The listing builds one solid part. Answer for the finished solid, in the listing's coordinates (mm). Coordinates: 2 decimals unless noted, no trailing zeros. Order: outer loops, then holes, each group sorted by start corner. A loop starts at its lowest first (then second) coordinate and runs counter-clockwise, first axis right, second up.
from build123d import *

# Parameters (mm, degrees)
ESBO_O1_R                  = 80
RESSALTO_EXTRUS_O1_DEPTH   = 5
CORTE_EXTRUS_O1_DEPTH      = 114.247516529
CORTE_EXTRUS_O1_DEPTH_BACK = 114.247516529
ESBO_O3_R                  = 6.75
CORTE_EXTRUS_O2_DEPTH      = 114.247516529
CORTE_EXTRUS_O2_DEPTH_BACK = 114.247516529
ESBO_O5_R                  = 4


with BuildPart() as part:
    # Esboço1 → Ressalto-extrusão1 (new body)
    with BuildSketch(Plane.XY):
        Circle(ESBO_O1_R)
    extrude(amount=RESSALTO_EXTRUS_O1_DEPTH)

    # Esboço3 → Corte-extrusão1 (cut, two sides: drawn at the far end of the back side and taken through both)
    with BuildSketch(Plane(origin=(0, 0, 0), x_dir=(-1, 0, 0), z_dir=(0, 0, -1)).offset(-CORTE_EXTRUS_O1_DEPTH_BACK)):
        with Locations((-15, 0)):
            Circle(ESBO_O3_R)
    extrude(amount=CORTE_EXTRUS_O1_DEPTH + CORTE_EXTRUS_O1_DEPTH_BACK, mode=Mode.SUBTRACT)

    # Esboço5 → Corte-extrusão2 (cut, two sides: drawn at the far end of the back side and taken through both)
    with BuildSketch(Plane(origin=(0, 0, 0), x_dir=(-1, 0, 0), z_dir=(0, 0, -1)).offset(-CORTE_EXTRUS_O2_DEPTH_BACK)):
        with Locations((23.941410033, 65.778483455)):
            Circle(ESBO_O5_R)
        with Locations((68.936542711, 12.155372437)):
            Circle(ESBO_O5_R)
        with Locations((44.995132678, -53.623111018)):
            Circle(ESBO_O5_R)
        with Locations((-23.941410033, -65.778483455)):
            Circle(ESBO_O5_R)
        with Locations((-68.936542711, -12.155372437)):
            Circle(ESBO_O5_R)
        with Locations((-44.995132678, 53.623111018)):
            Circle(ESBO_O5_R)
    extrude(amount=CORTE_EXTRUS_O2_DEPTH + CORTE_EXTRUS_O2_DEPTH_BACK, mode=Mode.SUBTRACT)


solid = part.part
1) Section D-D (y = 23.5) is taken. Give the vertices of the cut face in (x, z).
2) Each of these flat-tipped pins is pushed along its axis until it touches: P1, Ø1.5, axis at y = -6.5, z = 4, coming from the +X side; P2, Ø3, axis at y = -46, z = 3.5, coming from the +X side. Where does it stop, or does it pass through?
3) Consider L1, parallel to Y at x = 21, z = 3.15; L2, parallel to Y at x = 1.5, z = 3.85; L3, parallel to X at y = -13, z = 1.5. Determine where each line is inside the solid, lowest interval first.
4) Section C-C (z = 2.2) is taken. Give the vertices of the cut face in (x, y).
5) Determine the mould class of faces 1 (the face through (-17.34, -78.1, 2.46)), 2 (the face through (24.462, -61.813, 2.535)), 3 (the face through (-1, 1, 5)) for opening direction X: released by +X, released by -X, zero draft, split by the parting line, or undercut.
6) Section B-B (x = 15) is taken. Give the vertices of the cut face in (y, z), then the cut area to 3 significant figures.
7) Section A-A (y = 0) is taken. Give the vertices of the cut face in (x, z).
Filled sheet:
1. outline: (-76.47, 0) - (76.47, 0) - (76.47, 5) - (-76.47, 5) - close
2. P1: stops at x = 79.79
2. P2: stops at x = 66.48
3. L1: y = -77.19 to -68.49, -63.07 to -3.09, 3.09 to 77.19
3. L2: y = -79.99 to 79.99
3. L3: x = -78.94 to 65.03, 72.85 to 78.94
4. outline: circle Ø160 at (0, 0); hole circle Ø8 at (-68.94, 12.16); hole circle Ø8 at (-45, -53.62); hole circle Ø8 at (-23.94, 65.78); hole circle Ø13.5 at (15, 0); hole circle Ø8 at (23.94, -65.78); hole circle Ø8 at (45, 53.62); hole circle Ø8 at (68.94, -12.16)
5. face 1: split by the parting line
5. face 2: undercut
5. face 3: zero draft
6. outline: (-78.58, 0) - (-6.75, 0) - (-6.75, 5) - (-78.58, 5) - close; (6.75, 0) - (78.58, 0) - (78.58, 5) - (6.75, 5) - close
6. area: 718 mm2
7. outline: (-80, 0) - (8.25, 0) - (8.25, 5) - (-80, 5) - close; (21.75, 0) - (80, 0) - (80, 5) - (21.75, 5) - close
